Read the model definition and answer for the solid it produces. Units are mm, in the model's axes. Coordinates: 2 decimals unless noted, no trailing zeros. Loops run counter-clockwise (first coordinate to the right, second up) from the corner with the lowest first, then second, coordinate; pieces in that order, holes last. Notation, with made-up numbers: (-34, -39) -> (-24, -39) arc R8 ccw to (-24, -30) -> close; hole circle Ø4 at (5.5, 77). An arc over 180 degrees is marked (long way). Answer as a JSON object with one key per item and string values. Group by question number.
1) Section A-A, the plane y = -3 is taken. Give the vertices of the cut face in (x, z).
2) Section B-B, the plane z = 941 is taken. Give the vertices of the cut face in (x, y).
3) Section C-C, the plane x = 296 is taken. Give the vertices of the cut face in (y, z), plus the area to 3 significant figures.
4) Consider probe 1 along Z at (x, y) = (600, -10.5); probe 2 along X at (y, z) = (-7.5, 242.5); probe 3 along Z at (x, y) = (851.5, -5.25). Determine where each line is inside the solid, lowest interval first. Write a range as [from, to].
5) Flat-ended cylindrical pins translate along their axes: P1, Ø1.5, axis at x = 544.5, y = -11, coming from the -Z side; P2, Ø1.5, axis at x = 630.5, y = -13, coming from the -Z side; P3, Ø2, axis at y = -13, z = 597.5, coming from the +X side. Find the tip coordinate at first contact, or state that the pin passes through.
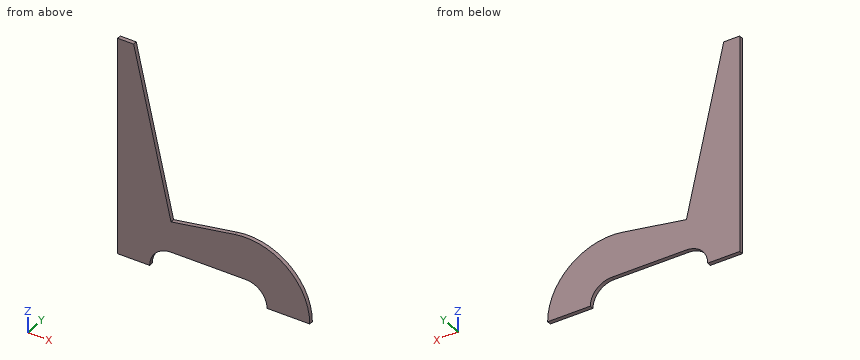
from build123d import *

# Parameters (mm, degrees)
F1_DEPTH = 19.05


with BuildPart() as f1:
    # F0 (on Front) → F1 (new body)
    with BuildSketch(Plane.XZ):
        with BuildLine():
            Line((0, 1041.4), (0, 0))
            Line((0, 0), (152.4, 0))
            ThreePointArc((152.4, 0), (182.157951, 71.842049), (254, 101.6))
            Line((254, 101.6), (609.6, 101.6))
            ThreePointArc((609.6, 101.6), (681.442049, 71.842049), (711.2, 0))
            Line((711.2, 0), (914.4, 0))
            ThreePointArc((914.4, 0), (806.075816, 233.024234), (558.09886, 300.417497))
            Line((558.09886, 300.417497), (254, 248.285254))
            Line((254, 248.285254), (76.2, 1041.4))
            Line((76.2, 1041.4), (0, 1041.4))
        make_face()
    extrude(amount=F1_DEPTH)


solid = f1.part
Determined:
{
 "1": {"outline": "(0, 0) -> (152.4, 0) arc R101.6 cw to (254, 101.6) -> (609.6, 101.6) arc R101.6 cw to (711.2, 0) -> (914.4, 0) arc R304.8 ccw to (558.1, 300.42) -> (254, 248.29) -> (76.2, 1041.4) -> (0, 1041.4) -> close"},
 "2": {"outline": "(0, -19.05) -> (98.71, -19.05) -> (98.71, 0) -> (0, 0) -> close"},
 "3": {"outline": "(-19.05, 101.6) -> (0, 101.6) -> (0, 255.49) -> (-19.05, 255.49) -> close", "area": "2,930 mm²"},
 "4": {"probe 1": "[101.6, 304.65]", "probe 2": "[0, 794.25]", "probe 3": "[0, 185.44]"},
 "5": {"P1": "z = 101.6", "P2": "z = 99.27", "P3": "x = 175.94"}
}
